```python
from build123d import *

# Parameters (mm, degrees)
F1_DEPTH = 25
F3_DEPTH = 8
F5_DEPTH = 8


with BuildPart() as f1:
    # F0 (on Front) → F1 (new body)
    with BuildSketch(Plane.XZ):
        Polygon((-40, -4), (40, -4), (40, 76), (32, 76), (32, 4), (-40, 4), align=None)
    extrude(amount=F1_DEPTH)

    # F2 (on face) → F3 (join)
    with BuildSketch(Plane(origin=(0, 0, 0), x_dir=(-1, 0, 0), z_dir=(0, 1, 0))):
        with BuildLine():
            Line((-32, 4), (40, 4))
            Line((40, 4), (40, 21))
            ThreePointArc((40, 21), (2.3807130871, 38.3807130871), (-15, 76))
            Line((-15, 76), (-32, 76))
            Line((-32, 76), (-32, 4))
        make_face()
    extrude(amount=-F3_DEPTH)

    # F4 (on face) → F5 (join)
    with BuildSketch(Plane.YZ.offset(40)):
        with BuildLine():
            Line((-80, -4), (-25, -4))
            Line((-25, -4), (-25, 76))
            ThreePointArc((-25, 76), (-41.1091270347, 37.1091270347), (-80, 21))
            Line((-80, 21), (-80, -4))
        make_face()
    extrude(amount=-F5_DEPTH)


solid = f1.part
```
Part model, mm, in its own coordinate system. A direction names the side the tool comes from. Give positions to 0.01 mm unless a question says otherwise; leave off trailing zeros. Order: outer loops, then holes, each group sorted by start corner. A loop starts at its lowest first (then second) coordinate and runs counter-clockwise, first axis right, second up. Notation, with made-up numbers: M -30,84 L -9,84 A10 cw -9,102 Z; hole C -32.75,56 d6. An arc over 180 degrees is marked long. Use a Markdown table: item, result. Add a question column.
(1) Saw through at B-B, the plane x = 35. Give the cut face in (y, z), and give its area (3 significant figures).
(2) Saw through at A-A, the plane z = 14. Give the cut face in (x, y), and give its area (3 significant figures).
(3) Probe line 1 along Z through (x, y) = (-23.5, -12); line 2 along Y through (x, z) = (25, 18.5); line 3 along X through (y, z) = (-48.5, 17). List the from-to ranges inside material, lowest first. Write a range as [from, to].
(4) Drop flat-ended pins along their axis: P1, Ø4, axis at x = 12.5, z = 1.5, coming from the -Y side; P2, Ø8.5, axis at x = 6.5, y = -17, coming from the +Z side; P3, Ø6, axis at x = -18.5, z = 30.5, coming from the +Y side; P4, Ø5, axis at x = 25.5, z = 21, coming from the +Y side. Give the stop position or say it passes through.
(5) 3-axis set-ups, long thin cutter, end or side, ignore diameter. For faces 4 (the face through (-40, -10, 3)), 5 (the face through (-5, -25, 0)), 6 (the face through (-3, -16, 4)): which of +Z, -Z, +X, -X, +Y, -Y reach the whole face in a straight line?
(6) Saw through at D-D, the plane y = -30.5. Give the cut face in (x, z), and give its area (3 significant figures).
(7) Mould opens along Z. For faces 1 (the face through (9, -23, -4)), 2 (the face through (36.056, -40.684, 37.539)), 3 (the face through (5, -8, 33)) say: +Z half, -Z half, draft (parallel to the pull), parting line (faces both ways), or undercut.
(8) Saw through at C-C, the plane y = -19. Give the cut face in (x, z).
Answer key:
| question | item | result |
|---|---|---|
| 1 | outline | M -80,-4 L 0,-4 L 0,76 L -25,76 A55 cw -80,21 Z |
| 1 | area | 4,020 mm^2 |
| 2 | outline | M -40,-8 L 32,-8 L 32,-80 L 40,-80 L 40,0 L -40,0 Z |
| 2 | area | 1,220 mm^2 |
| 3 | line 1 | [-4, 4] |
| 3 | line 2 | [-8, 0] |
| 3 | line 3 | [32, 40] |
| 4 | P1 | y = -25 |
| 4 | P2 | z = 4 |
| 4 | P3 | through |
| 4 | P4 | y = 0 |
| 5 | face 4 | +Z, -Z, -X, +Y, -Y |
| 5 | face 5 | +Z, -Z, -X, -Y |
| 5 | face 6 | +Z, -X, -Y |
| 6 | outline | M 32,-4 L 40,-4 L 40,52.03 L 32,52.03 Z |
| 6 | area | 448 mm^2 |
| 7 | face 1 | -Z half |
| 7 | face 2 | +Z half |
| 7 | face 3 | draft |
| 8 | outline | M -40,-4 L 40,-4 L 40,76 L 32,76 L 32,4 L -40,4 Z |
